Can you work these out from the model? Positions are in its coordinate system, mm. Face numbers are marked on the shaded views. A direction names the side the tool comes from. Give positions to 0.01 mm unless a question says otherwise; leave off trailing zeros. Write each loop counter-clockwise with the first axis right and the second up, starting at its lowest first coordinate (ties: lowest second). Pieces come first, ordered by that corner, then holes.
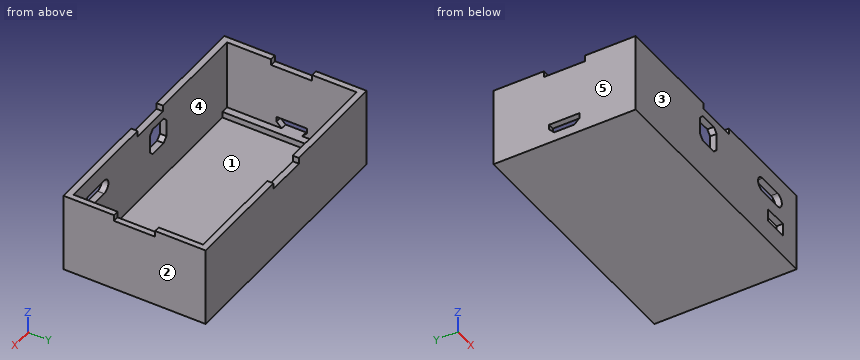
from build123d import *

# Parameters (mm, degrees)
CROQUIS1_W              = 58.2
CROQUIS1_H              = 31.7
CROQUIS1_R              = 1.55
SALIENTE_EXTRUIR1_DEPTH = 0.75
CROQUIS3_W              = 63
CROQUIS3_H              = 34.7
CROQUIS3_W_2            = 58.2
CROQUIS3_H_2            = 31.7
SALIENTE_EXTRUIR2_DEPTH = 2.25
CROQUIS4_W              = 63
CROQUIS4_H              = 34.7
CROQUIS4_W_2            = 60
CROQUIS4_H_2            = 31.619362532
SALIENTE_EXTRUIR3_DEPTH = 9.35
CROQUIS5_W              = 0.932931466
CROQUIS5_H              = 31.619362532
CORTAR_EXTRUIR1_DEPTH   = 10
CROQUIS6_W              = 0.932931466
CROQUIS6_H              = 31.619362532
SALIENTE_EXTRUIR4_DEPTH = 0.75
CROQUIS7_W              = 6.3
CROQUIS7_H              = 3.1
CORTAR_EXTRUIR2_DEPTH   = 10
CROQUIS9_W              = 63
CROQUIS9_H              = 34.7
CROQUIS9_W_2            = 60.1
CROQUIS9_H_2            = 31.619362532
SALIENTE_EXTRUIR5_DEPTH = 10
CROQUIS10_W             = 6.5
CROQUIS10_H             = 6.5
CORTAR_EXTRUIR3_DEPTH   = 10
CORTAR_EXTRUIR4_DEPTH   = 10
CROQUIS12_W             = 0.4
CROQUIS12_H             = 3.1
SALIENTE_EXTRUIR6_DEPTH = 1.580637468
CORTAR_EXTRUIR5_DEPTH   = 10
SALIENTE_EXTRUIR7_DEPTH = 1.580637468
CROQUIS15_W             = 63
CROQUIS15_H             = 34.7
SALIENTE_EXTRUIR8_DEPTH = 0.75
CORTAR_EXTRUIR6_DEPTH   = 1.5
CORTAR_EXTRUIR8_DEPTH   = 10
SALIENTE_EXTRUIR9_DEPTH = 1.5
CORTAR_EXTRUIR9_DEPTH   = 10


with BuildPart() as part:
    # Croquis1 → Saliente-Extruir1 (new body)
    with BuildSketch(Plane.XY):
        with Locations((5.077191095, -8.199822064)):
            Rectangle(CROQUIS1_W, CROQUIS1_H)
        with Locations((-20.872808905, 4.450177936)):
            Circle(CROQUIS1_R, mode=Mode.SUBTRACT)
        with Locations((31.027191095, 4.450177936)):
            Circle(CROQUIS1_R, mode=Mode.SUBTRACT)
        with Locations((-20.872808905, -20.849822064)):
            Circle(CROQUIS1_R, mode=Mode.SUBTRACT)
        with Locations((31.027191095, -20.849822064)):
            Circle(CROQUIS1_R, mode=Mode.SUBTRACT)
    extrude(amount=SALIENTE_EXTRUIR1_DEPTH)

    # Croquis3 → Saliente-Extruir2 (add)
    with BuildSketch(Plane(origin=(0, 0, 0), x_dir=(-1, 0, 0), z_dir=(0, 0, -1))):
        with Locations((-4.177191095, -8.199822064)):
            Rectangle(CROQUIS3_W, CROQUIS3_H)
        with Locations((-5.077191095, -8.199822064)):
            Rectangle(CROQUIS3_W_2, CROQUIS3_H_2, mode=Mode.SUBTRACT)
    extrude(amount=-SALIENTE_EXTRUIR2_DEPTH)

    # Croquis4 → Saliente-Extruir3 (add)
    with BuildSketch(Plane.XY):
        with Locations((4.177191095, -8.199822064)):
            Rectangle(CROQUIS4_W, CROQUIS4_H)
        with Locations((4.177191095, -8.15950333)):
            Rectangle(CROQUIS4_W_2, CROQUIS4_H_2, mode=Mode.SUBTRACT)
    extrude(amount=SALIENTE_EXTRUIR3_DEPTH)

    # Croquis5 → Cortar-Extruir1 (cut)
    with BuildSketch(Plane.XY):
        with Locations((33.810725362, -8.15950333)):
            Rectangle(CROQUIS5_W, CROQUIS5_H)
    extrude(amount=CORTAR_EXTRUIR1_DEPTH, mode=Mode.SUBTRACT)

    # Croquis6 → Saliente-Extruir4 (add)
    with BuildSketch(Plane(origin=(0, 0, 0), x_dir=(-1, 0, 0), z_dir=(0, 0, -1))):
        with Locations((-33.810725362, -8.15950333)):
            Rectangle(CROQUIS6_W, CROQUIS6_H)
    extrude(amount=-SALIENTE_EXTRUIR4_DEPTH)

    # Croquis7 → Cortar-Extruir2 (cut)
    with BuildSketch(Plane(origin=(0, -23.969184596, 0), x_dir=(1, 0, 0), z_dir=(0, 1, 0))):
        with Locations((27.127191095, -6.8)):
            Rectangle(CROQUIS7_W, CROQUIS7_H)
    extrude(amount=-CORTAR_EXTRUIR2_DEPTH, mode=Mode.SUBTRACT)

    # Croquis9 → Saliente-Extruir5 (add)
    with BuildSketch(Plane.XY.offset(9.35)):
        with Locations((4.177191095, -8.199822064)):
            Rectangle(CROQUIS9_W, CROQUIS9_H)
        with Locations((4.227191095, -8.15950333)):
            Rectangle(CROQUIS9_W_2, CROQUIS9_H_2, mode=Mode.SUBTRACT)
    extrude(amount=SALIENTE_EXTRUIR5_DEPTH)

    # Croquis10 → Cortar-Extruir3 (cut)
    with BuildSketch(Plane(origin=(0, -23.969184596, 0), x_dir=(1, 0, 0), z_dir=(0, 1, 0))):
        with Locations((1.127191095, -12.6)):
            Rectangle(CROQUIS10_W, CROQUIS10_H)
    extrude(amount=-CORTAR_EXTRUIR3_DEPTH, mode=Mode.SUBTRACT)

    # Croquis11 → Cortar-Extruir4 (cut)
    with BuildSketch(Plane(origin=(0, -23.969184596, 0), x_dir=(1, 0, 0), z_dir=(0, 1, 0))):
        with BuildLine():
            Line((22.277191095, -11.7), (28.177191095, -11.7))
            ThreePointArc((28.177191095, -11.7), (29.777191095, -13.3), (28.177191095, -14.9))
            Line((28.177191095, -14.9), (22.277191095, -14.9))
            ThreePointArc((22.277191095, -14.9), (20.677191095, -13.3), (22.277191095, -11.7))
        make_face()
    extrude(amount=-CORTAR_EXTRUIR4_DEPTH, mode=Mode.SUBTRACT)

    # Croquis12 → Saliente-Extruir6 (add)
    with BuildSketch(Plane.XZ.offset(25.549822064)):
        with Locations((24.177191095, 6.8)):
            Rectangle(CROQUIS12_W, CROQUIS12_H)
    extrude(amount=-SALIENTE_EXTRUIR6_DEPTH)

    # Croquis13 → Cortar-Extruir5 (cut)
    with BuildSketch(Plane(origin=(-25.822808905, 0, 0), x_dir=(0, 0, -1), z_dir=(1, 0, 0))):
        Polygon((-6.25, -4.434822064), (-5, -4.434822064), (-3.75, -5.684822064), (-3.75, -10.634822064), (-5, -11.884822064), (-6.25, -11.884822064), align=None)
    extrude(amount=-CORTAR_EXTRUIR5_DEPTH, mode=Mode.SUBTRACT)

    # Croquis14 → Saliente-Extruir7 (add)
    with BuildSketch(Plane.XZ.offset(25.549822064)):
        Polygon((4.377191095, 10.45), (3.277191095, 9.35), (4.377191095, 9.35), align=None)
        Polygon((-1.022808905, 9.35), (-2.122808905, 10.45), (-2.122808905, 9.35), align=None)
        Polygon((-2.122808905, 14.75), (-1.022808905, 15.85), (-2.122808905, 15.85), align=None)
        Polygon((3.277191095, 15.85), (4.377191095, 14.75), (4.377191095, 15.85), align=None)
    extrude(amount=-SALIENTE_EXTRUIR7_DEPTH)

    # Croquis15 → Saliente-Extruir8 (add)
    with BuildSketch(Plane(origin=(0, 0, 0), x_dir=(-1, 0, 0), z_dir=(0, 0, -1))):
        with Locations((-4.177191095, -8.199822064)):
            Rectangle(CROQUIS15_W, CROQUIS15_H)
    extrude(amount=-SALIENTE_EXTRUIR8_DEPTH)

    # Croquis16 → Cortar-Extruir6 (cut)
    with BuildSketch(Plane.XY.offset(19.35)):
        Polygon((-32.290822341, -3.199822064), (-0.822808905, -3.199822064), (-0.822808905, 14.947745762), (9.177191095, 14.947745762), (9.177191095, -3.199822064), (49.10392573, -3.199822064), (49.10392573, -13.199822064), (9.177191095, -13.199822064), (9.177191095, -34.683452232), (-0.822808905, -34.683452232), (-0.822808905, -13.199822064), (-32.290822341, -13.199822064), align=None)
    extrude(amount=-CORTAR_EXTRUIR6_DEPTH, mode=Mode.SUBTRACT)

    # Croquis17 → Cortar-Extruir8 (cut)
    with BuildSketch(Plane.XZ.offset(25.549822064)):
        with BuildLine():
            Line((22.277191095, 15), (28.177191095, 15))
            ThreePointArc((28.177191095, 15), (29.877191095, 13.3), (28.177191095, 11.6))
            Line((28.177191095, 11.6), (22.277191095, 11.6))
            ThreePointArc((22.277191095, 11.6), (20.577191095, 13.3), (22.277191095, 15))
        make_face()
    extrude(amount=-CORTAR_EXTRUIR8_DEPTH, mode=Mode.SUBTRACT)

    # Croquis22 → Saliente-Extruir9 (add)
    with BuildSketch(Plane.ZY.offset(27.322808905)):
        Polygon((6.25, -4.434822064), (6.25, -11.884822064), (5, -11.884822064), (3.75, -10.634822064), (3.75, -5.684822064), (5, -4.434822064), align=None)
    extrude(amount=-SALIENTE_EXTRUIR9_DEPTH)

    # Croquis24 → Cortar-Extruir9 (cut)
    with BuildSketch(Plane(origin=(-25.822808905, 0, 0), x_dir=(0, 0, -1), z_dir=(1, 0, 0))):
        Polygon((-2.25, -5.684822064), (-2.25, -10.634822064), (-3.501579003, -11.886401067), (-4.751579003, -11.886401067), (-4.751579003, -4.433243061), (-3.501579003, -4.433243061), align=None)
    extrude(amount=-CORTAR_EXTRUIR9_DEPTH, mode=Mode.SUBTRACT)


solid = part.part
(1) Will this pin go through, and if not, where does the flat tip stop? P1, Ø1.2, axis at x = 5.5, y = 8, coming from the +Z side.
Returned:
P1: stops at z = 17.85
(2) Imagine slicing it at B-B, the plane x = 5.5. Write out the boundary of the cut face in (y, z).
Returned:
outline: (-25.55, 0) - (9.15, 0) - (9.15, 17.85) - (7.65, 17.85) - (7.65, 0.75) - (-23.97, 0.75) - (-23.97, 17.85) - (-25.55, 17.85) - close
(3) If we mould it in two halves opening along Y, with no side actions, what happens to the marked faces 1, 2 and 3? For each: +Y half, -Y half, draft (parallel to the pull), parting line (faces both ways), or undercut.
Returned:
face 1: undercut
face 2: draft
face 3: -Y half
(4) Imagine slicing it at D-D, the plane y = -1. Write out the boundary of the cut face in (x, z).
Returned:
outline: (-27.32, 0) - (35.68, 0) - (35.68, 19.35) - (34.28, 19.35) - (34.28, 0.75) - (-24.02, 0.75) - (-24.02, 2.25) - (-25.82, 2.25) - (-25.82, 19.35) - (-27.32, 19.35) - close
(5) If I drill on L1, parallel to X at y = -7.5, z = 11.75; L2, parallel to Y at x = 22.5, z = 11; L3, parallel to Z at x = 28.5, y = 6, over which ranges is the centre line in solid material (lowest first)?
Returned:
L1: x = -27.32 to -25.82, 34.28 to 35.68
L2: y = -25.55 to -23.97, 7.65 to 9.15
L3: z = 0 to 0.75
(6) For the marked faces 4 and 5, which set-ups out of +Z, -Z, +X, -X, +Y, -Y let a thin tool reach every point of the face, with its end or its side?
Returned:
face 4: +Z
face 5: +Z, -Z, -X, +Y, -Y
(7) Imagine slicing it at A-A, the plane z = 13.3. Write out the boundary of the cut face in (x, y), plus the area to 3 significant figures.
Returned:
outline: (-27.32, -25.55) - (-2.12, -25.55) - (-2.12, -23.97) - (-25.82, -23.97) - (-25.82, 7.65) - (34.28, 7.65) - (34.28, -23.97) - (29.88, -23.97) - (29.88, -25.55) - (35.68, -25.55) - (35.68, 9.15) - (-27.32, 9.15) - close; (4.38, -25.55) - (20.58, -25.55) - (20.58, -23.97) - (4.38, -23.97) - close
area: 261 mm2
(8) Imagine slicing it at C-C, the plane z = 7.25. Write out the boundary of the cut face in (x, y).
Returned:
outline: (-27.32, -25.55) - (24.38, -25.55) - (24.38, -23.97) - (-25.82, -23.97) - (-25.82, 7.65) - (34.28, 7.65) - (34.28, -23.97) - (30.28, -23.97) - (30.28, -25.55) - (35.68, -25.55) - (35.68, 9.15) - (-27.32, 9.15) - close
